from build123d import *

# Parameters (mm, degrees)
BOSS_EXTRU_1_DEPTH    = 35
TROU_TARAUD_M31_D     = 2.5
TROU_TARAUD_M31_DEPTH = 4.9
TROU_TARAUD_M31_TIP   = 0.751075774
TROU_TARAUD_M32_D     = 2.5
TROU_TARAUD_M32_DEPTH = 4.9
TROU_TARAUD_M32_TIP   = 0.751075774


with BuildPart() as part:
    # Esquisse1 → Boss.-Extru.1 (new body)
    with BuildSketch(Plane.XY):
        Polygon((0, 0), (0, 12), (3, 12), (3, 3), (20, 3), (20, 0), align=None)
    extrude(amount=BOSS_EXTRU_1_DEPTH)

    # Trou taraudé M31
    with Locations(Plane(origin=(0, 3, 0), x_dir=(-1, 0, 0), z_dir=(0, 1, 0))):
        with Locations((-13.25, 27.824573519), (-13.25, 7.175426481)):
            Hole(TROU_TARAUD_M31_D / 2, depth=TROU_TARAUD_M31_DEPTH)
            with Locations((0, 0, -(TROU_TARAUD_M31_DEPTH + TROU_TARAUD_M31_TIP / 2))):  # 118° drill point
                Cone(0, TROU_TARAUD_M31_D / 2, TROU_TARAUD_M31_TIP, mode=Mode.SUBTRACT)

    # Trou taraudé M32
    with Locations(Plane.ZY):
        with Locations((6.786751346, 6), (28.013248654, 6)):
            Hole(TROU_TARAUD_M32_D / 2, depth=TROU_TARAUD_M32_DEPTH)
            with Locations((0, 0, -(TROU_TARAUD_M32_DEPTH + TROU_TARAUD_M32_TIP / 2))):  # 118° drill point
                Cone(0, TROU_TARAUD_M32_D / 2, TROU_TARAUD_M32_TIP, mode=Mode.SUBTRACT)


solid = part.part
Geometry: final body of the model. Coordinates: model frame, mm. A direction names the side the tool comes from. Give positions to 0.01 mm unless a question says otherwise; leave off trailing zeros. Loops run counter-clockwise (first coordinate to the right, second up) from the corner with the lowest first, then second, coordinate; pieces in that order, holes last. Notation, with made-up numbers: M 73.25,76 L 84.25,76 A3 cw 84.25,80 Z; hole C 34,-38.75 d7. An arc over 180 degrees is marked long. Put each result on its own line as item: value. Start each with the question number.
1) Ray query, line 1 along Y through (x, z) = (4.75, 21). Return the intervals inside material, ascending.
2) Pull-direction query (Z, two-part tool) for faces 3 (the flat face through (8, 2, 0)), 4 (the flat face through (20, 2, 17)), 5 (the cylindrical face through (13, 1.5, 26.6)); classes: pulls with the +Z half, pulls with the -Z half, needs draft (parallel to the pull), parting line crosses it, or undercut.
3) Cut plane D-D (x = 5.25). Output: boundary loops of the cut face in (y, z).
4) Cut plane B-B (y = 6). Output: boundary loops of the cut face in (x, z), then the cut area to 3 significant figures.
5) Cut plane A-A (x = 13.25). Output: boundary loops of the cut face in (y, z), then the cut area to 3 significant figures.
6) Access query for faces 1 (the flat face through (3, 8, 17)), 2 (the flat face through (1, 12, 17)). Directions: +Z, -Z, +X, -X, +Y, -Y. A direction counts if a zero-diameter tool reaches every point of the face in a straight line with its end or side. Return the directions, or none.
7) Contact query for flat-ended pins moving along their axis: pin 1 (8.5 mm diameter, centred on x = 14, z = 11, fed in from +Y); pin 2 (3 mm diameter, centred on y = 6, z = 6.79, fed in from +X); pin 3 (4 mm diameter, centred on x = 13.25, z = 27.82, fed in from -Y). Output: stop coordinate, or through.
8) Cut plane C-C (z = 17). Output: boundary loops of the cut face in (x, y).
Verdict:
1. line 1: 0 to 3
2. face 3: pulls with the -Z half
2. face 4: needs draft
2. face 5: undercut
3. outline: M 0,0 L 3,0 L 3,35 L 0,35 Z
4. outline: M 0,0 L 3,0 L 3,5.54 L 0,5.54 Z; M 0,8.04 L 3,8.04 L 3,26.76 L 0,26.76 Z; M 0,29.26 L 3,29.26 L 3,35 L 0,35 Z
4. area: 90.0 mm2
5. outline: M 0,0 L 3,0 L 3,5.93 L 0,5.93 Z; M 0,8.43 L 3,8.43 L 3,26.57 L 0,26.57 Z; M 0,29.07 L 3,29.07 L 3,35 L 0,35 Z
5. area: 90.0 mm2
6. face 1: +Z, -Z, +X, +Y
6. face 2: +Z, -Z, +X, -X, +Y
7. pin 1: y = 3
7. pin 2: x = 3
7. pin 3: y = 0
8. outline: M 0,0 L 20,0 L 20,3 L 3,3 L 3,12 L 0,12 Z
